Work out the finished part from the listing and answer in its coordinate system (mm). A direction names the side the tool comes from. Round coordinates to 2 decimals unless told otherwise and drop trailing zeros. Order: outer loops, then holes, each group sorted by start corner. A loop starts at its lowest first (then second) coordinate and runs counter-clockwise, first axis right, second up. Notation, with made-up numbers: (-13, -2.5) -> (2, -2.5) arc R13 ccw to (2, 2.5) -> close; hole circle Ø10 at (89.25, -5.5). An arc over 180 degrees is marked (long way). Use a Markdown table: item, result. Add a question column.
Item 1: Flat-ended cylindrical pins translate along their axes: P1, Ø4.5, axis at x = 8, z = -15.5, coming from the -Y side; P2, Ø3.5, axis at x = -8, z = -15.5, coming from the +Y side; P3, Ø5, axis at x = 7, y = 0, coming from the -Z side. Find the tip coordinate at first contact, or state that the pin passes through.
Item 2: A cutting plane is placed at B-B, the plane y = -7. Determine the outline of the cut face in (x, z), plus the area to 3 significant figures.
Item 3: A cutting plane is placed at D-D, the plane x = 7. Determine the outline of the cut face in (y, z).
Item 4: A tool of negligible diameter and unlimited length cuts with its end or side. For faces 1 (the flat face through (0, 28, -14)), 2 (the cylindrical face through (6.373, 37.535, -16.747)), 3 (the cylindrical face through (-0.325, 5.536, 3.944)), from which of +Z, -Z, +X, -X, +Y, -Y can it reach the whole face along a straight path? Write none if from no direction.
Item 5: For a pull along Z with two mould halves and no side action, classify faces 4 (the flat face through (0, 34, -24)), 5 (the flat face through (8, 35, -15)), 6 (the cylindrical face through (0, -12, 4)), 7 (the flat face through (-8, 35, -15)) as +Z half, -Z half, draft (parallel to the pull), parting line (faces both ways), or undercut.
Item 6: A cutting plane is placed at A-A, the plane x = 0. Determine the outline of the cut face in (y, z), plus the area to 4 significant figures.
Item 7: Find the intervals of material crossed by L1, parallel to Z at x = -8, y = 37; L2, parallel to Y at x = 0, z = 2.5; L3, parallel to Z at x = -1, y = 5, in increasing order. Write a range as [from, to].
Item 8: A cutting plane is placed at C-C, the plane y = 0. Determine the outline of the cut face in (x, z).
from build123d import *

# Parameters (mm, degrees)
SKETCH1_R           = 1.5
BOSS_EXTRUDE1_DEPTH = 8
BOSS_EXTRUDE2_DEPTH = 24
CHAMFER1_SIZE       = 5
CUT_EXTRUDE2_REACH  = 10
SKETCH5_R           = 3
SKETCH6_R           = 2.05
CUT_EXTRUDE6_DEPTH  = 5


with BuildPart() as part:
    # Sketch1 → Boss-Extrude1 (new body)
    with BuildSketch(Plane.XY):
        with BuildLine():
            Line((-16, 40), (-11.942152172, -1.176860869))
            ThreePointArc((-11.942152172, -1.176860869), (0, -12), (11.942152172, -1.176860869))
            Line((11.942152172, -1.176860869), (16, 40))
            Line((16, 40), (-16, 40))
        make_face()
        with Locations((7, 0)):
            Circle(SKETCH1_R, mode=Mode.SUBTRACT)
        with Locations((0, 7)):
            Circle(SKETCH1_R, mode=Mode.SUBTRACT)
        with Locations((0, -7)):
            Circle(SKETCH1_R, mode=Mode.SUBTRACT)
        with Locations((-7, 0)):
            Circle(SKETCH1_R, mode=Mode.SUBTRACT)
    extrude(amount=BOSS_EXTRUDE1_DEPTH)

    # Sketch3 → Boss-Extrude2 (add)
    with BuildSketch(Plane(origin=(0, 0, 0), x_dir=(-1, 0, 0), z_dir=(0, 0, -1))):
        Polygon((14.817438413, 28), (-14.817438413, 28), (-16, 40), (16, 40), align=None)
    extrude(amount=BOSS_EXTRUDE2_DEPTH)

    # Chamfer1
    chamfer1_edges = [part.edges().sort_by_distance(p)[0] for p in [
        (0, 28, 0),
    ]]
    chamfer(chamfer1_edges, length=CHAMFER1_SIZE)

    # Sketch5 → Cut-Extrude2 (cut, up to next)
    with BuildSketch(Plane(origin=(0, 0, 0), x_dir=(-1, 0, 0), z_dir=(0, 0, -1)), mode=Mode.PRIVATE) as cut_extrude2_sk1:
        Circle(SKETCH5_R)
    cut_extrude2_tool1 = extrude(cut_extrude2_sk1.sketch, amount=-CUT_EXTRUDE2_REACH, mode=Mode.PRIVATE) & part.part
    add(cut_extrude2_tool1.solids().sort_by_distance((0, 0, 0))[0], mode=Mode.SUBTRACT)

    # Sketch6 → Cut-Extrude6 (cut)
    with BuildSketch(Plane.XZ.offset(-40)):
        with Locations((-8, -15.5)):
            Circle(SKETCH6_R)
        with Locations((8, -15.5)):
            Circle(SKETCH6_R)
    extrude(amount=CUT_EXTRUDE6_DEPTH, mode=Mode.SUBTRACT)


solid = part.part
Reported:
| question | item | result |
|---|---|---|
| 1 | P1 | y = 28 |
| 1 | P2 | y = 35 |
| 1 | P3 | z = 0 |
| 2 | outline | (-9.75, 0) -> (-1.5, 0) -> (-1.5, 8) -> (-9.75, 8) -> close; (1.5, 0) -> (9.75, 0) -> (9.75, 8) -> (1.5, 8) -> close |
| 2 | area | 132 mm² |
| 3 | outline | (-9.75, 0) -> (-1.5, 0) -> (-1.5, 8) -> (-9.75, 8) -> close; (1.5, 0) -> (23, 0) -> (28, -5) -> (28, -24) -> (40, -24) -> (40, -17.29) -> (35, -17.29) -> (35, -13.71) -> (40, -13.71) -> (40, 8) -> (1.5, 8) -> close |
| 4 | face 1 | -Z, +X, -X, -Y |
| 4 | face 2 | +Y |
| 4 | face 3 | +Z, -Z |
| 5 | face 4 | -Z half |
| 5 | face 5 | undercut |
| 5 | face 6 | draft |
| 5 | face 7 | undercut |
| 6 | outline | (-12, 0) -> (-8.5, 0) -> (-8.5, 8) -> (-12, 8) -> close; (-5.5, 0) -> (-3, 0) -> (-3, 8) -> (-5.5, 8) -> close; (3, 0) -> (5.5, 0) -> (5.5, 8) -> (3, 8) -> close; (8.5, 0) -> (23, 0) -> (28, -5) -> (28, -24) -> (40, -24) -> (40, 8) -> (8.5, 8) -> close |
| 6 | area | 620.5 mm² |
| 7 | L1 | [-24, -17.55], [-13.45, 8] |
| 7 | L2 | [-12, -8.5], [-5.5, -3], [3, 5.5], [8.5, 40] |
| 7 | L3 | [0, 8] |
| 8 | outline | (-12.06, 0) -> (-8.5, 0) -> (-8.5, 8) -> (-12.06, 8) -> close; (-5.5, 0) -> (-3, 0) -> (-3, 8) -> (-5.5, 8) -> close; (3, 0) -> (5.5, 0) -> (5.5, 8) -> (3, 8) -> close; (8.5, 0) -> (12.06, 0) -> (12.06, 8) -> (8.5, 8) -> close |
